Design review of the part built by this model. Coordinates are the model's own, in mm. A direction names the side the tool comes from. Coordinates: 2 decimals unless noted, no trailing zeros. Order: outer loops, then holes, each group sorted by start corner. A loop starts at its lowest first (then second) coordinate and runs counter-clockwise, first axis right, second up.
from build123d import *

# Parameters (mm, degrees)
SKETCH2_R           = 1.75
BOSS_EXTRUDE1_DEPTH = 6
CHAMFER1_SIZE       = 0.5


with BuildPart() as part:
    # Sketch2 → Boss-Extrude1 (new body)
    with BuildSketch(Plane(origin=(0, 0, 0), x_dir=(1, 0, 0), z_dir=(0, 1, 0))):
        with BuildLine():
            Line((11, 2.2), (15, 2.2))
            ThreePointArc((15, 2.2), (18.25, -1.05), (15, -4.3))
            Line((15, -4.3), (0, -4.3))
            Line((0, -4.3), (0, 0))
            Line((0, 0), (11, 0))
            Line((11, 0), (11, 2.2))
        make_face()
        with Locations(Location((15, -1.05, 0), (0, 0, 270))):
            Circle(SKETCH2_R, mode=Mode.SUBTRACT)
    extrude(amount=BOSS_EXTRUDE1_DEPTH)

    # Chamfer1
    chamfer1_edges = [part.edges().sort_by_distance(p)[0] for p in [
        (15, 6, -0.7),
    ]]
    chamfer(chamfer1_edges, length=CHAMFER1_SIZE)


solid = part.part
1. Mouldability with a two-part tool opening along X and no side actions: class faces 3 (the flat face through (11, 3, -1)), 4 (the flat face through (9, 6, 2)), 5 (the cylindrical face through (16.735, 2.712, 0.822)), 6 (the cylindrical face through (18.25, 2.96, 0.98)) as pulls with the +X half, pulls with the -X half, needs draft (parallel to the pull), parting line crosses it, or undercut.
2. Add section C-C (x = 1.5). Give the boundary of the cut face in (y, z), and give its area (3 significant figures).
3. To check wall thickness, follow line 1 (X direction, y = 3.1, z = 1.05); line 2 (X direction, y = 5.75, z = 0.5); line 3 (Z direction, x = 14.5, y = 3.4). State the ranges of each line that lie inside material, in increasing order.
4. Add section D-D (z = -1.5). Give the boundary of the cut face in (x, y), and give its area (3 significant figures).
5. Add section B-B (y = 1.85). Give the boundary of the cut face in (x, z).
6. Add section A-A (z = 1.05). Give the boundary of the cut face in (x, y).
7. Insertion check: pin 1 (1.5 mm diameter, centred on x = 16, y = 3, fed in from +Z); pin 2 (3 mm diameter, centred on y = 4, z = 3, fed in from +X); pin 3 (1.8 mm diameter, centred on y = 4, z = -1, fed in from -X). Each pin has a flat end and moves straight along its axis. Give the tip position at first contact, or say it passes through.
8. For faces 1 (the flat face through (8, 3, 4.3)), 2 (the flat face through (5, 3, 0)), list the 3-axis set-ups (+Z, -Z, +X, -X, +Y, -Y) from which the entire face can be reached by the end or side of a thin tool; tool diameter is ignored.
Solution:
1. face 3: pulls with the -X half
1. face 4: needs draft
1. face 5: undercut
1. face 6: pulls with the +X half
2. outline: (0, 0) - (6, 0) - (6, 4.3) - (0, 4.3) - close
2. area: 25.8 mm2
3. line 1: x = 0 to 13.25, 16.75 to 18.25
3. line 2: x = 0 to 13.08, 16.92 to 18.2
3. line 3: z = -2.2 to -0.63, 2.73 to 4.3
4. outline: (11, 0) - (17.01, 0) - (17.01, 6) - (11, 6) - close
4. area: 36.1 mm2
5. outline: (0, 0) - (11, 0) - (11, -2.2) - (15, -2.2) arc R3.25 ccw to (15, 4.3) - (0, 4.3) - close; hole circle Ø3.5 at (15, 1.05)
6. outline: (0, 0) - (13.25, 0) - (13.25, 5.5) - (12.75, 6) - (0, 6) - close; (16.75, 0) - (18.25, 0) - (18.25, 6) - (17.25, 6) - (16.75, 5.5) - close
7. pin 1: stops at z = 4.29
7. pin 2: stops at x = 18.22
7. pin 3: stops at x = 11
8. face 1: +Z, +X, -X, +Y, -Y
8. face 2: -Z, -X, +Y, -Y
